The listing builds one solid part. Answer for the finished solid, in the listing's coordinates (mm). Face numbers are marked on the shaded views. A direction names the side the tool comes from. Give positions to 0.01 mm unless a question says otherwise; leave off trailing zeros. Order: outer loops, then holes, each group sorted by start corner. A loop starts at its lowest first (then second) coordinate and runs counter-clockwise, first axis right, second up. Notation, with made-up numbers: (-9, -16) - (12, -16) arc R21 ccw to (12, 16) - close; hole circle Ø6 at (-10.5, 76.5). An arc over 180 degrees is marked (long way). Answer in a Markdown table with one row per item.
from build123d import *

# Parameters (mm, degrees)
SKETCH1_W               = 266
SKETCH1_H               = 156
BOSS_EXTRUDE1_DEPTH     = 10
SKETCH2_W               = 230
SKETCH2_H               = 80
BOSS_EXTRUDE2_DEPTH     = 60
FILLET1_R               = 90
FILLET2_R               = 20
CUT_EXTRUDE1_DEPTH      = 40
CUT_EXTRUDE1_DEPTH_BACK = 40
FILLET3_R               = 10
CUT_EXTRUDE2_REACH      = 225.886
SKETCH4_R               = 20
SKETCH5_W               = 69.5
SKETCH5_H               = 38.16369677
CUT_EXTRUDE3_DEPTH      = 18
SKETCH6_R               = 4
CUT_EXTRUDE4_DEPTH      = 179.530109674
FILLET4_R               = 30


with BuildPart() as part:
    # Sketch1 → Boss-Extrude1 (new body)
    with BuildSketch(Plane(origin=(0, 0, 0), x_dir=(1, 0, 0), z_dir=(0, 1, 0))):
        Rectangle(SKETCH1_W, SKETCH1_H)
    extrude(amount=BOSS_EXTRUDE1_DEPTH)

    # Sketch2 → Boss-Extrude2 (add, symmetric)
    with BuildSketch(Plane.XY):
        with Locations((0, 50)):
            Rectangle(SKETCH2_W, SKETCH2_H)
    extrude(amount=BOSS_EXTRUDE2_DEPTH, both=True)

    # Fillet1
    # the kernel refuses this fillet: 90 mm, written as the material it takes off along each edge
    with BuildSketch(Plane(origin=(-115, 90, -283.60679775), x_dir=(0, -1, 0), z_dir=(0, 0, 1))) as fillet1_piece_1:
        with BuildLine():
            CenterArc((90, 89.4427191), FILLET1_R, 180, 83.620629792)
            Line((0, 89.4427191), (-1.8, 89.4427191))
            Line((-1.8, 89.4427191), (-1.8, 0))
            Line((-1.8, 0), (0, -1.8))
            ThreePointArc((0, -1.8), (40, -1.8), (79.8, -1.788854382))
            Line((79.8, -1.788854382), (80, 0))
        make_face()
    extrude(amount=567.2135955, mode=Mode.SUBTRACT)

    # Fillet2
    fillet2_edges = [part.edges().sort_by_distance(p)[0] for p in [
        (115, 50, 60),
        (115, 90, 0),
        (115, 50, -60),
        (44.72135955, 90, -60),
        (-85.5572809, 67.082039325, -60),
        (44.72135955, 90, 60),
        (-85.5572809, 67.082039325, 60),
    ]]
    fillet(fillet2_edges, radius=FILLET2_R)

    # Sketch3 → Cut-Extrude1 (cut, two sides: drawn at the far end of the back side and taken through both)
    with BuildSketch(Plane.XY.offset(-CUT_EXTRUDE1_DEPTH_BACK)):
        with BuildLine():
            Line((-105.5572809, 0), (105, 0))
            Line((105, 0), (105, 60))
            ThreePointArc((105, 60), (99.142135624, 74.142135624), (85, 80))
            Line((85, 80), (-25.5572809, 80))
            ThreePointArc((-25.5572809, 80), (-82.125823395, 56.568542495), (-105.5572809, 0))
        make_face()
    extrude(amount=CUT_EXTRUDE1_DEPTH + CUT_EXTRUDE1_DEPTH_BACK, mode=Mode.SUBTRACT)

    # Fillet3
    fillet3_edges = [part.edges().sort_by_distance(p)[0] for p in [
        (99.142135624, 74.142135624, -40),
        (105, 30, -40),
        (-82.125823395, 56.568542495, -40),
        (29.72135955, 80, -40),
        (105, 30, 40),
        (99.142135624, 74.142135624, 40),
        (29.72135955, 80, 40),
        (-82.125823395, 56.568542495, 40),
    ]]
    fillet(fillet3_edges, radius=FILLET3_R)

    # Sketch4 → Cut-Extrude2 (cut, up to next)
    with BuildSketch(Plane(origin=(0, 0, -78), x_dir=(-1, 0, 0), z_dir=(0, 0, -1)), mode=Mode.PRIVATE) as cut_extrude2_sk1:
        with Locations((-5, -3)):
            Circle(SKETCH4_R)
    cut_extrude2_tool1 = extrude(cut_extrude2_sk1.sketch, amount=-CUT_EXTRUDE2_REACH, mode=Mode.PRIVATE) & part.part
    add(cut_extrude2_tool1.solids().sort_by_distance((5, -3, -78))[0], mode=Mode.SUBTRACT)

    # Sketch5 → Cut-Extrude3 (cut)
    with BuildSketch(Plane(origin=(0, 0, -78), x_dir=(-1, 0, 0), z_dir=(0, 0, -1))):
        with Locations((-5, 0)):
            Rectangle(SKETCH5_W, SKETCH5_H)
    extrude(amount=-CUT_EXTRUDE3_DEPTH, mode=Mode.SUBTRACT)

    # Sketch6 → Cut-Extrude4 (cut, through all)
    with BuildSketch(Plane.XZ):
        with Locations(Location((-125, -28, 0), (0, 0, 270))):
            Circle(SKETCH6_R)
        with Locations(Location((125, -28, 0), (0, 0, 270))):
            Circle(SKETCH6_R)
        with Locations(Location((125, 28, 0), (0, 0, 270))):
            Circle(SKETCH6_R)
        with Locations(Location((-125, 28, 0), (0, 0, 270))):
            Circle(SKETCH6_R)
        with Locations(Location((-73, -70, 0), (0, 0, 270))):
            Circle(SKETCH6_R)
        with Locations(Location((67, -70, 0), (0, 0, 270))):
            Circle(SKETCH6_R)
        with Locations(Location((-3, 70, 0), (0, 0, 270))):
            Circle(SKETCH6_R)
        with Locations(Location((67, 70, 0), (0, 0, 270))):
            Circle(SKETCH6_R)
        with Locations(Location((-73, 70, 0), (0, 0, 270))):
            Circle(SKETCH6_R)
    extrude(amount=-CUT_EXTRUDE4_DEPTH, mode=Mode.SUBTRACT)

    # Fillet4
    fillet4_edges = [part.edges().sort_by_distance(p)[0] for p in [
        (133, 5, 78),
        (-133, 5, 78),
        (-133, 5, -78),
        (133, 5, -78),
    ]]
    fillet(fillet4_edges, radius=FILLET4_R)


solid = part.part
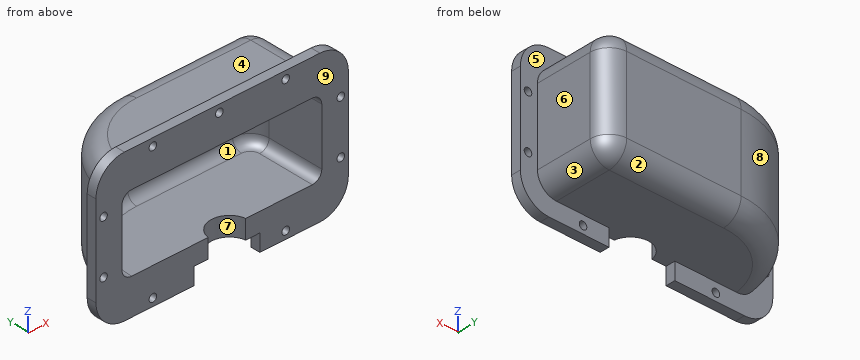
Item 1: Find section A-A on x = 67. Write down the section's boundary in (y, z).
Answer block:
| item | result |
|---|---|
| outline | (0, -78) - (10, -78) - (10, -74) - (0, -74) - close; (0, -66) - (10, -66) - (10, -60) - (70, -60) arc R20 ccw to (90, -40) - (90, 40) arc R20 ccw to (70, 60) - (10, 60) - (10, 66) - (0, 66) - (0, 40) - (70, 40) arc R10 cw to (80, 30) - (80, -30) arc R10 cw to (70, -40) - (0, -40) - close; (0, 74) - (10, 74) - (10, 78) - (0, 78) - close |
Item 2: Which of the six approach directions +Z, -Z, +X, -X, +Y, -Y give full straight-line access (tool end or side, diameter ignored) to the marked faces 1, 2, 3, 4 and 5?
Answer block:
| item | result |
|---|---|
| face 1 | -Y |
| face 2 | -Z, +X, -X, +Y |
| face 3 | -Z, +X, +Y |
| face 4 | +Z, +X, -X, +Y |
| face 5 | +Y |
Item 3: Find section C-C on z = 70. Write down the section's boundary in (x, y).
Answer block:
| item | result |
|---|---|
| outline | (-123.4, 0) - (-77, 0) - (-77, 10) - (-123.4, 10) - close; (-69, 0) - (-7, 0) - (-7, 10) - (-69, 10) - close; (1, 0) - (63, 0) - (63, 10) - (1, 10) - close; (71, 0) - (123.4, 0) - (123.4, 10) - (71, 10) - close |
Item 4: Each of these flat-tipped pins is pushed along its axis until it touches: P1, Ø3, axis at y = 46.5, z = -15, coming from the +X side; P2, Ø3, axis at x = -54, y = 74, coming from the -Z side; P3, Ø5, axis at y = 61, z = 57, coming from the -X side. Where does it stop, or does it pass through?
Answer block:
| item | result |
|---|---|
| P1 | x = 115 |
| P2 | z = -58.43 |
| P3 | x = -83.77 |
Item 5: Find section D-D on x = -10. Write down the section's boundary in (y, z).
Answer block:
| item | result |
|---|---|
| outline | (0, 40) - (70, 40) arc R10 cw to (80, 30) - (80, -30) arc R10 cw to (70, -40) - (10.23, -40) - (10.23, -60) - (70, -60) arc R20 ccw to (90, -40) - (90, 40) arc R20 ccw to (70, 60) - (10, 60) - (10, 78) - (0, 78) - close |
Item 6: Determine the mould class of the marked faces 6, 7, 8 and 9 for opening direction X: pulls with the +X half, pulls with the -X half, needs draft (parallel to the pull), parting line crosses it, or undercut.
Answer block:
| item | result |
|---|---|
| face 6 | pulls with the +X half |
| face 7 | undercut |
| face 8 | pulls with the -X half |
| face 9 | needs draft |
Item 7: Consider line 1 (X direction, y = 3, z = 28); line 2 (Z direction, x = 16.5, y = 14); line 3 (X direction, y = 6.25, z = 70). Determine where each line is inside the solid, lowest interval first.
Answer block:
| item | result |
|---|---|
| line 1 | -133 to -129, -121 to -105.5, 105 to 121, 129 to 133 |
| line 2 | -60 to -40, 40 to 60 |
| line 3 | -123.4 to -77, -69 to -7, 1 to 63, 71 to 123.4 |
Item 8: Find section B-B on z = 13. Write down the section's boundary in (x, y), then the cut area to 3 significant figures.
Answer block:
| item | result |
|---|---|
| outline | (-133, 0) - (-105.56, 0) arc R80 cw to (-25.56, 80) - (85, 80) arc R20 cw to (105, 60) - (105, 0) - (133, 0) - (133, 10) - (115, 10) - (115, 70) arc R20 ccw to (95, 90) - (-25.56, 90) arc R90 ccw to (-115, 10) - (-133, 10) - close |
| area | 3,900 mm² |
